Check sheet for the modelled part. Datum: model origin and axes. Units: mm. Face numbers are marked on the shaded views. A direction names the side the tool comes from. Give positions to 0.01 mm unless a question says otherwise; leave off trailing zeros. Loops run counter-clockwise (first coordinate to the right, second up) from the corner with the lowest first, then second, coordinate; pieces in that order, holes last. Notation, with made-up numbers: M 40,10.25 L 68,10.25 A28 cw 68,31.25 Z; hole C 32.5,-12 d2. An arc over 180 degrees is marked long. Write each question's results on one line, items separated by ' | '. Start each with the question number.
1. Sectioned sample at C-C on x = 13. Record the cut outline in (y, z) (3 decimals).
2. Material ranges on line 1 along Z through (x, y) = (39, 46); line 2 along Y through (x, z) = (44, -13.5); line 3 along Y through (x, z) = (32.5, -17), recorded low to high.
3. Tool access check on the marked faces 1 and 2. Record the directions out of +Z, -Z, +X, -X, +Y, -Y that give a thin tool (end or side, any length) a straight path to the whole face; none if there is none.
4. Go/stop test with flat-tipped pins: pin 1 (12 mm diameter, centred on x = 35.5, y = 39, fed in from +Z); pin 2 (0.6 mm diameter, centred on x = 41, y = -1, fed in from -Z); pin 3 (10 mm diameter, centred on x = 41.5, z = -7, fed in from +Y); pin 4 (2.5 mm diameter, centred on x = 14.29, y = 44.45, fed in from -Z). Record where each tip stops, or that it passes through.
5. Sectioned sample at D-D on y = 2.5. Record the cut outline in (x, z).
6. Sectioned sample at B-B on x = 31.5. Record the cut outline in (y, z) (3 decimals), and give its area (3 significant figures).
7. Sectioned sample at A-A on y = 44.45. Record the cut outline in (x, z), and give its area (3 significant figures).
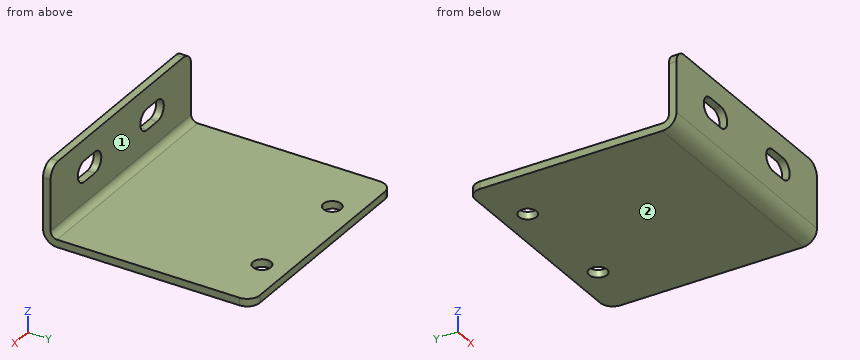
```python
from build123d import *

# Parameters (mm, degrees)
SKETCH1_W                      = 57.15
SKETCH1_H                      = 15.875
BASE_FLANGE1_DEPTH             = 1.89738
EDGE_FLANGE1_DEPTH             = 57.15
F_4_START                      = -1.89738
F_4_0_209_DIAMETER_SLOT1_DEPTH = 1.89738
F_4_5_4_5_DIAMETER_HOLE1_D     = 4.5
FILLET1_R                      = 3.175


# Read off the part's stored shape, not the designer's step: #4 (0.209) Diameter Slot1
# Sheet-metal steps are written as plain solids
with BuildPart() as part:
    # Sketch1 → Base-Flange1 (new body)
    with BuildSketch(Plane(origin=(0, 0, 0), x_dir=(1, 0, 0), z_dir=(0, 1, 0))):
        with Locations((28.575, 7.9375)):
            Rectangle(SKETCH1_W, SKETCH1_H)
    extrude(amount=-BASE_FLANGE1_DEPTH)

    # Edge-Flange1 section (across the edge) → Edge-Flange1 (add)
    with BuildSketch(Plane(origin=(57.15, 0, -17.526), x_dir=(0, 0, 1), z_dir=(-1, 0, 0))):
        with BuildLine():
            Line((-1.89738, 1.651), (-1.89738, 50.8))
            Line((-1.89738, 50.8), (0, 50.8))
            Line((0, 50.8), (0, 1.651))
            ThreePointArc((0, 1.651), (0.483566704, 0.483566704), (1.651, 0))
            Line((1.651, 0), (1.651, -1.89738))
            ThreePointArc((1.651, -1.89738), (-0.85808356, -0.85808356), (-1.89738, 1.651))
        make_face()
    extrude(amount=EDGE_FLANGE1_DEPTH)

    # #4 (0.209) Diameter Slot1 outline → #4 (0.209) Diameter Slot1 (cut)
    with BuildSketch(Plane(origin=(0, 0, 0), x_dir=(1, 0, 0), z_dir=(0, 1, 0)).offset(F_4_START)):
        with BuildLine():
            Line((39.1668, 5.2832), (43.3832, 5.2832))
            ThreePointArc((43.3832, 5.2832), (46.0375, 7.9375), (43.3832, 10.5918))
            Line((43.3832, 10.5918), (39.1668, 10.5918))
            ThreePointArc((39.1668, 10.5918), (36.5125, 7.9375), (39.1668, 5.2832))
        make_face()
        with BuildLine():
            ThreePointArc((17.9832, 5.2832), (20.6375, 7.9375), (17.9832, 10.5918))
            Line((17.9832, 10.5918), (13.7668, 10.5918))
            ThreePointArc((13.7668, 10.5918), (11.1125, 7.9375), (13.7668, 5.2832))
            Line((13.7668, 5.2832), (17.9832, 5.2832))
        make_face()
    extrude(amount=F_4_0_209_DIAMETER_SLOT1_DEPTH, mode=Mode.SUBTRACT)

    # Ø4.5 (4.5) Diameter Hole1 (through all)
    with Locations(Plane.XY.offset(-17.526)):
        with Locations((14.2875, 44.45), (42.8625, 44.45)):
            Hole(F_4_5_4_5_DIAMETER_HOLE1_D / 2)

    # Fillet1
    fillet1_edges = [part.edges().sort_by_distance(p)[0] for p in [
        (57.15, 50.8, -18.47469),
        (0, 50.8, -18.47469),
        (57.15, -0.94869, 0),
        (0, -0.94869, 0),
    ]]
    fillet(fillet1_edges, radius=FILLET1_R)


solid = part.part
```
Output values:
1) outline: M -1.897,-15.875 A3.548 ccw 1.651,-19.423 L 42.605,-19.423 L 42.605,-17.526 L 1.651,-17.526 A1.651 cw 0,-15.875 L 0,-10.479 L -1.897,-10.479 Z; M -1.897,-5.396 L 0,-5.396 L 0,0 L -1.897,0 Z; M 46.295,-19.423 L 50.8,-19.423 L 50.8,-17.526 L 46.295,-17.526 Z
2) line 1: -19.42 to -17.53 | line 2: -1.9 to 0 | line 3: -1.71 to 0.44
3) face 1: +Z, +X, -X, +Y | face 2: -Z, +X, -X, +Y, -Y
4) pin 1: z = -17.53 | pin 2: z = -18.53 | pin 3: y = 0 | pin 4: through
5) outline: M 0,-19.42 L 57.15,-19.42 L 57.15,-17.53 L 0,-17.53 Z
6) outline: M -1.897,-15.875 A3.548 ccw 1.651,-19.423 L 50.8,-19.423 L 50.8,-17.526 L 1.651,-17.526 A1.651 cw 0,-15.875 L 0,0 L -1.897,0 Z | area: 131 mm2
7) outline: M 0,-19.42 L 12.04,-19.42 L 12.04,-17.53 L 0,-17.53 Z; M 16.54,-19.42 L 40.61,-19.42 L 40.61,-17.53 L 16.54,-17.53 Z; M 45.11,-19.42 L 57.15,-19.42 L 57.15,-17.53 L 45.11,-17.53 Z | area: 91.4 mm2
